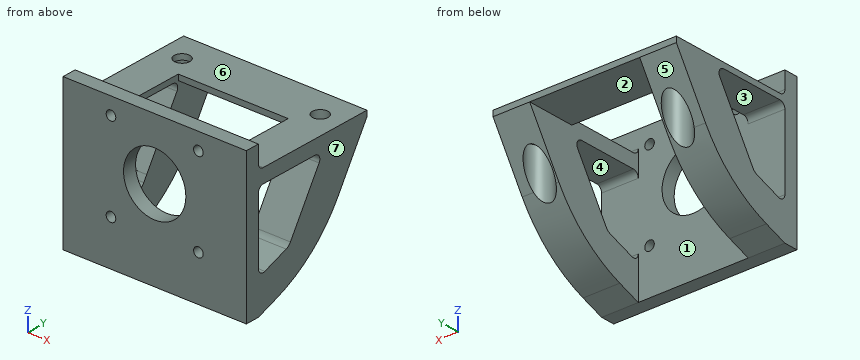
from build123d import *

# Parameters (mm, degrees)
BOSS_EXTRUDE1_DEPTH  = 32.5
SKETCH2_R            = 11.05
CUT_EXTRUDE1_DEPTH   = 43
SKETCH3_W            = 23
SKETCH3_H            = 90
CUT_EXTRUDE2_DEPTH   = 65.577472852
M5_CLEARANCE_HOLE1_D = 5.5
M3_CLEARANCE_HOLE1_D = 3.4
SKETCH9_W            = 8
SKETCH9_H            = 45
CUT_EXTRUDE3_DEPTH   = 4
SKETCH13_W           = 10
SKETCH13_H           = 5
BOSS_EXTRUDE4_DEPTH  = 65
BOSS_EXTRUDE5_START  = -13
BOSS_EXTRUDE5_DEPTH  = 13
SKETCH10_R           = 4.5
CUT_EXTRUDE4_DEPTH   = 71.215738976
BOSS_EXTRUDE6_START  = -13
BOSS_EXTRUDE6_DEPTH  = 13
FILLET1_R            = 2
SKETCH16_R           = 4.5
SKETCH16_R_2         = 2.75
BOSS_EXTRUDE7_DEPTH  = 5
SKETCH18_W           = 39
SKETCH18_H           = 17.431843069
BOSS_EXTRUDE8_DEPTH  = 2
SKETCH11_W           = 4
SKETCH11_H           = 14.485426666
CUT_EXTRUDE5_DEPTH   = 76.638945064


with BuildPart() as part:
    # Sketch1 → Boss-Extrude1 (new, symmetric)
    with BuildSketch(Plane(origin=(0, 0, 0), x_dir=(0, 0, -1), z_dir=(1, 0, 0))):
        Polygon((-11.5, 45), (-11.5, 0), (21.5, 0), (21.5, -5), (-21.5, -5), (-21.5, 0), (-13.5, 0), (-13.5, 45), align=None)
    extrude(amount=BOSS_EXTRUDE1_DEPTH, both=True)

    # Sketch2 → Cut-Extrude1 (cut)
    with BuildSketch(Plane.XZ.offset(5)):
        with Locations(Location((0, 0, 0), (0, 0, 270))):
            Circle(SKETCH2_R)
    extrude(amount=-CUT_EXTRUDE1_DEPTH, mode=Mode.SUBTRACT)

    # Sketch3 → Cut-Extrude2 (cut, through all)
    with BuildSketch(Plane(origin=(0, 0, 11.5), x_dir=(-1, 0, 0), z_dir=(0, 0, -1))):
        with Locations((0, 45)):
            Rectangle(SKETCH3_W, SKETCH3_H)
    extrude(amount=-CUT_EXTRUDE2_DEPTH, mode=Mode.SUBTRACT)

    # M5 Clearance Hole1 (through all)
    with Locations(Plane(origin=(0, 0, 11.5), x_dir=(-1, 0, 0), z_dir=(0, 0, -1))):
        with Locations((-24.5, 35), (24.5, 35)):
            Hole(M5_CLEARANCE_HOLE1_D / 2)

    # M3 Clearance Hole1 (through all)
    with Locations(Plane(origin=(0, -5, 0), x_dir=(-1, 0, 0), z_dir=(0, -1, 0))):
        with Locations((-15.5, 15.5), (15.5, 15.5), (15.5, -15.5), (-15.5, -15.5)):
            Hole(M3_CLEARANCE_HOLE1_D / 2)

    # Sketch9 → Cut-Extrude3 (cut)
    with BuildSketch(Plane(origin=(0, 0, 11.5), x_dir=(-1, 0, 0), z_dir=(0, 0, -1))):
        with Locations((-15.5, 22.5)):
            Rectangle(SKETCH9_W, SKETCH9_H)
    cut_extrude3 = extrude(amount=-CUT_EXTRUDE3_DEPTH, mode=Mode.SUBTRACT)

    # Mirror1: Cut-Extrude3 across plane
    add(cut_extrude3.mirror(Plane(origin=(0, 0, 0), x_dir=(0, 0, 1), z_dir=(1, 0, 0))), mode=Mode.SUBTRACT)

    # Sketch13 → Boss-Extrude4 (add)
    with BuildSketch(Plane.ZY.offset(32.5)):
        with Locations((-26.5, -2.5)):
            Rectangle(SKETCH13_W, SKETCH13_H)
    extrude(amount=-BOSS_EXTRUDE4_DEPTH)

    # Sketch14 → Boss-Extrude5 (add)
    with BuildSketch(Plane.ZY.offset(32.5).offset(BOSS_EXTRUDE5_START)):
        with BuildLine():
            Line((-19.5, 0), (-15.318472481, 11.488652437))
            ThreePointArc((-15.318472481, 11.488652437), (-14.742301187, 12.503177188), (-13.864717431, 13.271994839))
            Line((-13.864717431, 13.271994839), (11.5, 28.893048142))
            Line((11.5, 28.893048142), (11.5, 45))
            Line((11.5, 45), (-8.132103018, 32.909420693))
            ThreePointArc((-8.132103018, 32.909420693), (-20.553998297, 22.027072107), (-28.709504164, 7.666824297))
            Line((-28.709504164, 7.666824297), (-31.5, 0))
            Line((-31.5, 0), (-19.5, 0))
        make_face()
    boss_extrude5 = extrude(amount=BOSS_EXTRUDE5_DEPTH)

    # Mirror4: Boss-Extrude5 across plane
    add(boss_extrude5.mirror(Plane(origin=(0, 0, 0), x_dir=(0, 0, 1), z_dir=(1, 0, 0))))

    # Sketch10 → Cut-Extrude4 (cut, through all)
    with BuildSketch(Plane(origin=(0, 0, 11.5), x_dir=(-1, 0, 0), z_dir=(0, 0, -1))):
        with Locations(Location((-24.5, 35, 0), (0, 0, 207.682602444))):
            Circle(SKETCH10_R)
    cut_extrude4 = extrude(amount=CUT_EXTRUDE4_DEPTH, mode=Mode.SUBTRACT)

    # Mirror3: Cut-Extrude4 across plane
    add(cut_extrude4.mirror(Plane(origin=(0, 0, 0), x_dir=(0, 0, 1), z_dir=(1, 0, 0))), mode=Mode.SUBTRACT)

    # Sketch15 → Boss-Extrude6 (add)
    with BuildSketch(Plane(origin=(32.5, 0, 0), x_dir=(0, 0, -1), z_dir=(1, 0, 0)).offset(BOSS_EXTRUDE6_START)):
        Polygon((-11.5, 0), (-8.5, 0), (-8.5, 27.045475425), (-11.5, 28.893048142), align=None)
    extrude(amount=BOSS_EXTRUDE6_DEPTH)

    # Fillet1
    fillet1_edges = [part.edges().sort_by_distance(p)[0] for p in [
        (-26, 0, 11.5),
        (-26, 0, 13.5),
        (26, 0, 13.5),
        (-26, 0, -19.5),
        (-26, 28.893048142, 11.5),
        (26, 0, -19.5),
        (26, 27.045475425, 8.5),
        (26, 0, 8.5),
    ]]
    fillet(fillet1_edges, radius=FILLET1_R)

    # Sketch16 → Boss-Extrude7 (add)
    with BuildSketch(Plane(origin=(0, 0, 11.5), x_dir=(-1, 0, 0), z_dir=(0, 0, -1))):
        with Locations(Location((-24.5, 35, 0), (0, 0, 207.682602444))):
            Circle(SKETCH16_R)
        with Locations(Location((-24.5, 35, 0), (0, 0, 90))):
            Circle(SKETCH16_R_2, mode=Mode.SUBTRACT)
    boss_extrude7 = extrude(amount=BOSS_EXTRUDE7_DEPTH)

    # Mirror5: Boss-Extrude7 across plane
    add(boss_extrude7.mirror(Plane(origin=(0, 0, 0), x_dir=(0, 0, 1), z_dir=(1, 0, 0))))

    # Sketch18 → Boss-Extrude8 (add)
    with BuildSketch(Plane.XY.offset(13.5)):
        with Locations((0, 36.284078466)):
            Rectangle(SKETCH18_W, SKETCH18_H)
    extrude(amount=-BOSS_EXTRUDE8_DEPTH)

    # Mirror2: Cut-Extrude4 across plane
    add(cut_extrude4.mirror(Plane(origin=(0, 0, 0), x_dir=(0, 0, 1), z_dir=(1, 0, 0))), mode=Mode.SUBTRACT)

    # Sketch11 → Cut-Extrude5 (cut, through all)
    with BuildSketch(Plane(origin=(-19.5, 0, 0), x_dir=(0, 0, -1), z_dir=(1, 0, 0))):
        with Locations((9.900667288, 7.242713333)):
            Rectangle(SKETCH11_W, SKETCH11_H)
    extrude(amount=-CUT_EXTRUDE5_DEPTH, mode=Mode.SUBTRACT)


solid = part.part
Build history of the part. All positions in model axes, mm. Face numbers are marked on the shaded views. A direction names the side the tool comes from. Coordinates: 2 decimals unless noted, no trailing zeros. Write each loop counter-clockwise with the first axis right and the second up, starting at its lowest first coordinate (ties: lowest second). Pieces come first, ordered by that corner, then holes.
(1) 3-axis set-ups, long thin cutter, end or side, ignore diameter. For the marked faces 1, 2 and 3: which of +Z, -Z, +X, -X, +Y, -Y reach the whole face in a straight line?
(2) Pin check, flat tips, straight feed: pin 1 Ø13 at (x, y) = (-11.5, 32.5) entering from +Z; pin 2 Ø2.5 at (x, z) = (15.5, 15.5) entering from +Y; pin 3 Ø4 at (x, y) = (28.5, 12) entering from -Z; pin 4 Ø10 at (x, z) = (11, -7.5) entering from +Y. Stop position of each tip, or through.
(3) Cut at A-A on x = 0. List the corners of the cut face in (y, z), and give its area (3 significant figures).
(4) Cut at C-C on y = 35. List the corners of the cut face in (x, z), and give its area (3 significant figures).
(5) Drill centre lines: line 1 (X direction, y = -2.75, z = -15.5); line 2 (X direction, y = 35, z = -4.25); line 3 (Z direction, x = -15.5, y = -3.65). Where is each one in solid material? Low to high.
(6) Cut at B-B on x = 15.5. List the corners of the cut face in (y, z).
(7) Cut at D-D on x = -24.5. State how many separate pieces and enclosed holes the cut face has, and give its area (3 significant figures).
(8) Mould opens along Z. For the marked faces 4, 5, 6 and 7 say: pulls with the +Z half, pulls with the -Z half, needs draft (parallel to the pull), parting line crosses it, or undercut.
Working result:
1. face 1: none
1. face 2: -Z, +Y
1. face 3: -X
2. pin 1: stops at z = 13.5
2. pin 2: passes through
2. pin 3: stops at z = -27.79
2. pin 4: stops at y = 0
3. outline: (-5, -31.5) - (0, -31.5) - (0, -11.05) - (-5, -11.05) - close; (-5, 11.05) - (0, 11.05) - (0, 21.5) - (-5, 21.5) - close; (27.57, 11.5) - (45, 11.5) - (45, 13.5) - (27.57, 13.5) - close
3. area: 189 mm2
4. outline: (-32.5, -4.74) - (-29, -4.74) - (-29, 11.5) - (-27.25, 11.5) - (-27.25, 13.5) - (-32.5, 13.5) - close; (-21.75, 11.5) - (-20, 11.5) - (-20, -4.74) - (-19.5, -4.74) - (-19.5, 11.5) - (19.5, 11.5) - (19.5, -4.74) - (20, -4.74) - (20, 6.5) - (21.75, 6.5) - (21.75, 13.5) - (-21.75, 13.5) - close; (27.25, 6.5) - (29, 6.5) - (29, -4.74) - (32.5, -4.74) - (32.5, 13.5) - (27.25, 13.5) - close
4. area: 255 mm2
5. line 1: x = -32.5 to -17.2, -13.8 to 13.8, 17.2 to 32.5
5. line 2: x = -32.5 to -29, -20 to -19.5, 19.5 to 20, 29 to 32.5
5. line 3: z = -31.5 to -17.2, -13.8 to 13.8, 17.2 to 21.5
6. outline: (-5, -31.5) - (0, -31.5) - (0, -17.2) - (-5, -17.2) - close; (-5, -13.8) - (0, -13.8) - (0, 13.8) - (-5, 13.8) - close; (-5, 17.2) - (0, 17.2) - (0, 21.5) - (-5, 21.5) - close; (27.57, 11.5) - (45, 11.5) - (45, 13.5) - (27.57, 13.5) - close
7. separate pieces: 2
7. enclosed holes: 1
7. area: 881 mm2
8. face 4: undercut
8. face 5: pulls with the -Z half
8. face 6: pulls with the +Z half
8. face 7: needs draft
